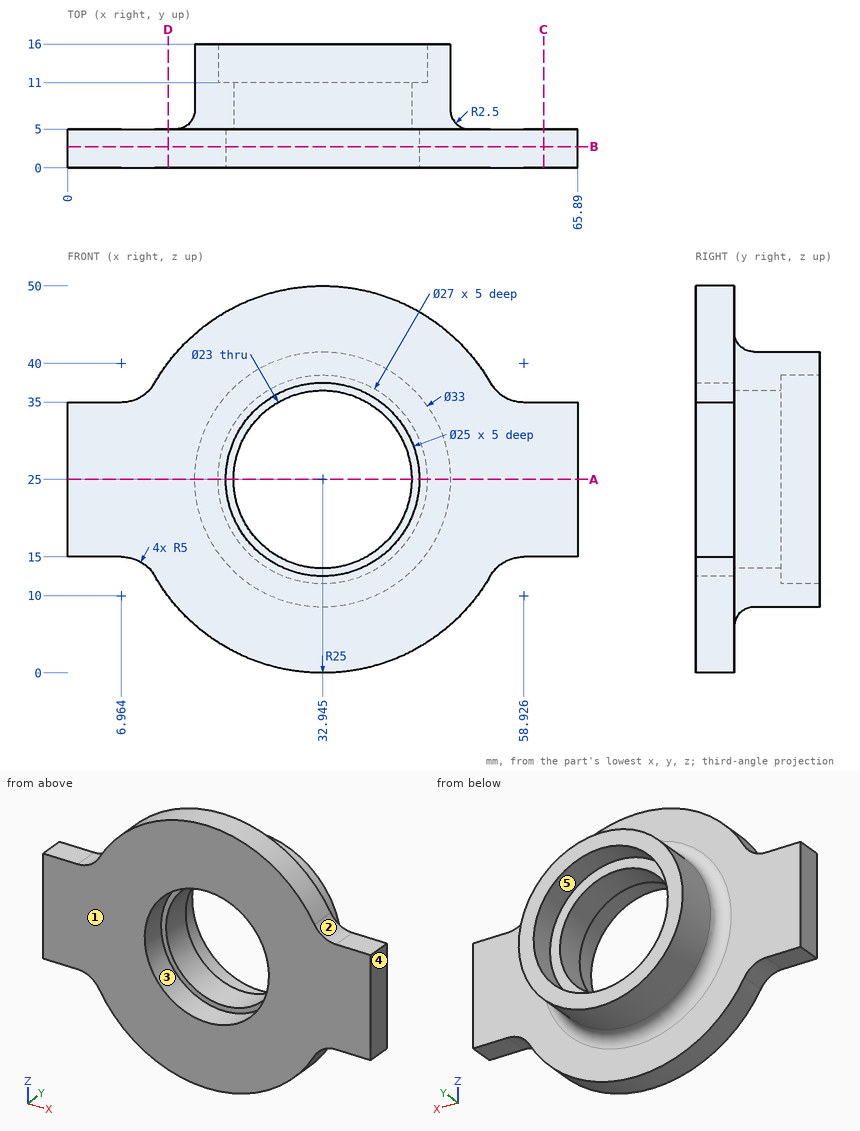
Can you work these out from the drawing? Everything is in mm from the part's minimum corner. A direction names the side the tool comes from. Round coordinates to 2 decimals unless told otherwise and drop trailing zeros. Write each loop counter-clockwise with the first axis right and the second up, starting at its lowest first coordinate (ties: lowest second). Pieces come first, ordered by that corner, then holes. Notation, with made-up numbers: (33, 23.25) - (73, 23.25) arc R27 cw to (73, 43.25) - close; hole circle Ø11 at (88.25, 21). An arc over 180 degrees is marked (long way). Use a Markdown table: item, result.
Q1. Thinking about a two-plate mould opening in X: for the marked faces 1, 2 and 3, which applies, released by +X, released by -X, zero draft, split by the parting line, or undercut?
Output values:
| item | result |
|---|---|
| face 1 | zero draft |
| face 2 | released by +X |
| face 3 | undercut |
Q2. I want a section at A-A (z = 25). List the corners of the cut face in (x, y) for me (3 decimals), plus the area to 3 significant figures.
Output values:
| item | result |
|---|---|
| outline | (0, 0) - (20.445, 0) - (20.445, 5) - (21.445, 5) - (21.445, 11) - (19.445, 11) - (19.445, 16) - (16.445, 16) - (16.445, 7.5) arc R2.5 cw to (13.945, 5) - (0, 5) - close; (44.445, 5) - (45.445, 5) - (45.445, 0) - (65.89, 0) - (65.89, 5) - (51.945, 5) arc R2.5 cw to (49.445, 7.5) - (49.445, 16) - (46.445, 16) - (46.445, 11) - (44.445, 11) - close |
| area | 297 mm2 |
Q3. I want a section at D-D (x = 13). List the corners of the cut face in (y, z) for me.
Output values:
| item | result |
|---|---|
| outline | (0, 9.93) - (5, 9.93) - (5, 40.07) - (0, 40.07) - close |
Q4. For pin 1 (4 mm diameter, centred on x = 62.5, y = 1.5, fed in from +Z); pin 2 (6 mm diameter, centred on x = 58, y = 3.5, fed in from -Z); pin 3 (5 mm diameter, centred on x = 35.5, z = 5.5, fed in from +Y), each with a flat end and sliding along its axis, tell me the tip position at first contact or that it passes through.
Output values:
| item | result |
|---|---|
| pin 1 | z = 35 |
| pin 2 | z = 13.1 |
| pin 3 | y = 5.8 |
Q5. I want a section at C-C (x = 61.5). List the corners of the cut face in (y, z) for me.
Output values:
| item | result |
|---|---|
| outline | (0, 15) - (5, 15) - (5, 35) - (0, 35) - close |
Q6. Please list where these lines run through material, in increasing order: L1, parallel to X at y = 13, z = 25 (3 decimals); L2, parallel to X at y = 9.05, z = 25 (3 decimals); L3, parallel to Y at x = 29, z = 5.5.
Output values:
| item | result |
|---|---|
| L1 | 16.445 to 19.445, 46.445 to 49.445 |
| L2 | 16.445 to 21.445, 44.445 to 49.445 |
| L3 | 0 to 5 |
Q7. For the marked faces 4 and 5, which set-ups out of +Z, -Z, +X, -X, +Y, -Y let a thin tool reach every point of the face, with its end or its side?
Output values:
| item | result |
|---|---|
| face 4 | +Z, -Z, +X, +Y, -Y |
| face 5 | +Y |
Q8. I want a section at B-B (y = 2.75). List the corners of the cut face in (x, z) for me (1 decimal).
Output values:
| item | result |
|---|---|
| outline | (0, 15) - (7, 15) arc R5 cw to (11.3, 12.5) arc R25 ccw to (54.6, 12.5) arc R5 cw to (58.9, 15) - (65.9, 15) - (65.9, 35) - (58.9, 35) arc R5 cw to (54.6, 37.5) arc R25 ccw to (11.3, 37.5) arc R5 cw to (7, 35) - (0, 35) - close; hole circle Ø25 at (32.9, 25) |
